Job drawing, mm, ordinate dimensions from the low corner. One solid piece. A direction names the side the tool comes from. Round coordinates to 2 decimals unless told otherwise and drop trailing zeros. Loops run counter-clockwise (first coordinate to the right, second up) from the corner with the lowest first, then second, coordinate; pieces in that order, holes last. Notation, with made-up numbers: M 30.5,89 L 36.5,89 A23 ccw 36.5,119 Z; hole C 41,72.5 d10. An arc over 180 degrees is marked long. Use a Markdown table: item, result. Add a question column.
(1) Flat gauge pins, fed straight in: P1, Ø12, axis at y = 77.5, z = 77, coming from the -X side; P2, Ø12, axis at x = 129, y = 96, coming from the +Z side. Where does each tip first touch, or does it go through?
(2) Wall check: L1, parallel to X at y = 44, z = 9; L2, parallel to X at y = 97, z = 94; L3, parallel to Y at x = 107.95, z = 18. Give the ranges that are in metal, low to high.
(3) Band-saw the part on D-D, the plane z = 48. Write the cut outline in (x, y), and give its area (3 significant figures).
(4) Which spindle directions (+Z, -Z, +X, -X, +Y, -Y) get a long thin tool onto all of the face, cutting with end or side? Do the marked faces 4, 5, 6, 7 and 8. Say none if no direction does.
(5) Band-saw the part on B-B, the plane y = 44.45. Write the cut outline in (x, z).
(6) Band-saw the part on C-C, the plane x = 107.95. Write the cut outline in (y, z), and give its area (3 significant figures).
(7) Band-saw the part on A-A, the plane z = 74. Write the cut outline in (x, y).
(8) Two-plate mould, pull along X, no slides. Class the marked faces 1, 2 and 3: released by +X, released by -X, zero draft, split by the parting line, or undercut.
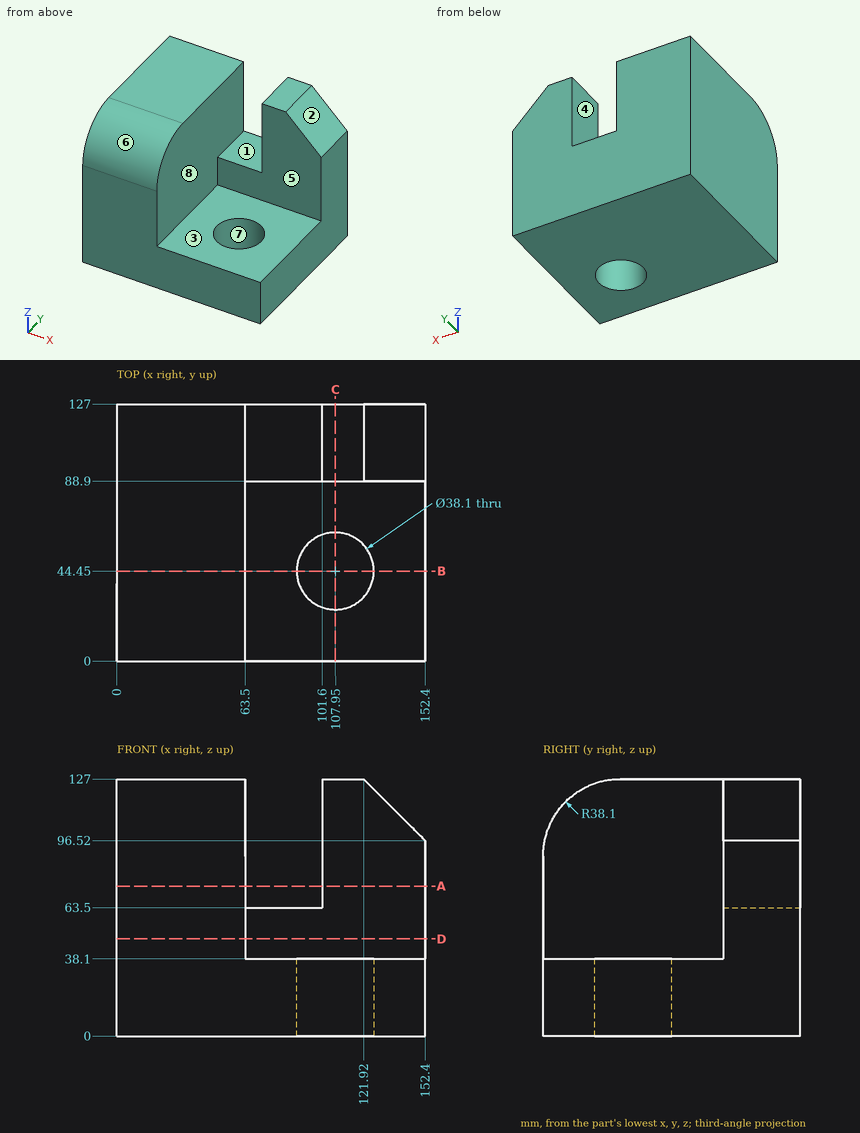
Return value:
| question | item | result |
|---|---|---|
| 1 | P1 | x = 0 |
| 1 | P2 | z = 125.92 |
| 2 | L1 | 0 to 88.91, 126.99 to 152.4 |
| 2 | L2 | 0 to 63.5, 101.6 to 152.4 |
| 2 | L3 | 0 to 25.4, 63.5 to 127 |
| 3 | outline | M 0,0 L 63.5,0 L 63.5,88.9 L 152.4,88.9 L 152.4,127 L 0,127 Z |
| 3 | area | 11,500 mm^2 |
| 4 | face 4 | +Z, +Y, -Y |
| 4 | face 5 | +Z, +X, -Y |
| 4 | face 6 | +Z, +X, -X, -Y |
| 4 | face 7 | +Z, -Z |
| 4 | face 8 | +Z, -Y |
| 5 | outline | M 0,0 L 88.9,0 L 88.9,38.1 L 63.5,38.1 L 63.5,127 L 0,127 Z; M 127,0 L 152.4,0 L 152.4,38.1 L 127,38.1 Z |
| 6 | outline | M 0,0 L 25.4,0 L 25.4,38.1 L 0,38.1 Z; M 63.5,0 L 127,0 L 127,127 L 88.9,127 L 88.9,38.1 L 63.5,38.1 Z |
| 6 | area | 6,770 mm^2 |
| 7 | outline | M 0,0 L 63.5,0 L 63.5,127 L 0,127 Z; M 101.6,88.9 L 152.4,88.9 L 152.4,127 L 101.6,127 Z |
| 8 | face 1 | undercut |
| 8 | face 2 | released by +X |
| 8 | face 3 | zero draft |
